from build123d import *

# Parameters (mm, degrees)
SKETCH2_W           = 12.139554842
SKETCH2_H           = 17.312906794
BOSS_EXTRUDE1_DEPTH = 15.24
SKETCH3_R           = 7.354852585
BOSS_EXTRUDE2_DEPTH = 1.27
SKETCH4_R           = 7.343962116
BOSS_EXTRUDE3_DEPTH = 19.05
FILLET1_R           = 5.08
FILLET2_R           = 2.54
SKETCH5_R           = 2.9177626
BOSS_EXTRUDE4_DEPTH = 13.97
BOSS_EXTRUDE5_DEPTH = 3.81
FILLET3_R           = 2.54
SKETCH8_R           = 1.866604038
CUT_EXTRUDE1_DEPTH  = 54.61
FILLET4_R           = 2.54


with BuildPart() as part:
    # Sketch1 → Revolve1 (revolve)
    with BuildSketch(Plane(origin=(0, 0, 0), x_dir=(1, 0, 0), z_dir=(0, 1, 0))):
        Polygon((0, 0), (-25.668765954, 0), (-37.871949768, 49.023134977), (-35.374465572, 49.023134977), (-23.974578156, 3.227035533), (0, 3.227035533), align=None)
    revolve(axis=Axis((0, 0, -3.227035533), (0, 0, 1)))

    # Sketch2 → Boss-Extrude1 (add)
    with BuildSketch(Plane.XY):
        Rectangle(SKETCH2_W, SKETCH2_H)
    extrude(amount=BOSS_EXTRUDE1_DEPTH)

    # Sketch3 → Boss-Extrude2 (add)
    with BuildSketch(Plane(origin=(0, 8.656453397, 0), x_dir=(1, 0, 0), z_dir=(0, 1, 0))):
        with Locations((0, -6.679713392)):
            Circle(SKETCH3_R)
    extrude(amount=BOSS_EXTRUDE2_DEPTH)

    # Sketch4 → Boss-Extrude3 (add)
    with BuildSketch(Plane.XZ.offset(-8.656453397)):
        with Locations((0.010679396, 6.67757966)):
            Circle(SKETCH4_R)
    extrude(amount=BOSS_EXTRUDE3_DEPTH)

    # Fillet1
    fillet1_edges = [part.edges().sort_by_distance(p)[0] for p in [
        (23.974578156, 0, -3.227035533),
    ]]
    fillet(fillet1_edges, radius=FILLET1_R)

    # Fillet2
    fillet2_edges = [part.edges().sort_by_distance(p)[0] for p in [
        (25.668765954, 0, 0),
    ]]
    fillet(fillet2_edges, radius=FILLET2_R)

    # Sketch5 → Boss-Extrude4 (add)
    with BuildSketch(Plane.XY.offset(15.24)):
        Circle(SKETCH5_R)
    extrude(amount=BOSS_EXTRUDE4_DEPTH)

    # Sketch6 → Boss-Extrude5 (add)
    with BuildSketch(Plane.XY.offset(15.24)):
        Polygon((1.022367717, -3.695378883), (3.711475848, -0.962293026), (2.689108131, 2.733085857), (-1.022367717, 3.695378883), (-3.711475848, 0.962293026), (-2.689108131, -2.733085857), align=None)
    extrude(amount=BOSS_EXTRUDE5_DEPTH)

    # Fillet3
    # the kernel refuses this fillet: 2.54 mm, written as the material it adds along each edge
    with BuildSketch(Plane(origin=(6.069777421, -8.656453397, 2.527747051), x_dir=(0, 0, -1), z_dir=(0, 1, 0))) as fillet3_piece_1:
        with BuildLine():
            CenterArc((0.723381963, -2.54), FILLET3_R, 90, 29.540761072)
            ThreePointArc((-0.52894629, -0.330186898), (-0.260967221, -0.170709801), (0, 0))
            Line((0, 0), (0.723381963, 0))
        make_face()
    extrude(amount=17.312906794)
    with BuildSketch(Plane(origin=(6.069777421, -8.656453397, 10.827412269), x_dir=(0.5295323324681384, 0, -0.8482897552551564), z_dir=(0, 1, 0))) as fillet3_piece_2:
        with BuildLine():
            CenterArc((0.731374616, -2.537710116), FILLET3_R, 92.433100789, 29.540761072)
            Line((-0.613637508, -0.383054138), (0, 0))
            ThreePointArc((0, 0), (0.311772179, -0.006620794), (0.623544358, 0))
        make_face()
    extrude(amount=17.312906794)
    with BuildSketch(Plane(origin=(-6.069777421, -8.656453397, 10.796053219), x_dir=(-0.5254687488151466, 0, -0.8508129018877444), z_dir=(0, 1, 0))) as fillet3_piece_3:
        with BuildLine():
            CenterArc((0.724778579, 2.537751252), FILLET3_R, 238.300195445, 29.288660156)
            Line((-0.609912043, 0.376686481), (0, 0))
            ThreePointArc((0, 0), (0.308960404, 0.006501859), (0.617920808, 0))
        make_face()
    extrude(amount=17.312906794)
    with BuildSketch(Plane(origin=(-6.069777421, -8.656453397, 2.559106101), x_dir=(-0.5254687488151472, 0, 0.8508129018877438), z_dir=(0, 1, 0))) as fillet3_piece_4:
        with BuildLine():
            CenterArc((0.724778579, -2.537751252), FILLET3_R, 92.411144399, 29.288660156)
            Line((-0.609912043, -0.376686481), (0, 0))
            ThreePointArc((0, 0), (0.308960404, -0.006501859), (0.617920808, 0))
        make_face()
    extrude(amount=17.312906794)

    # Sketch8 → Cut-Extrude1 (cut)
    with BuildSketch(Plane(origin=(0, 0, -3.227035533), x_dir=(-1, 0, 0), z_dir=(0, 0, -1))):
        Circle(SKETCH8_R)
    extrude(amount=-CUT_EXTRUDE1_DEPTH, mode=Mode.SUBTRACT)

    # Fillet4
    fillet4_edges = [part.edges().sort_by_distance(p)[0] for p in [
        (1.866604038, 0, -3.227035533),
    ]]
    fillet(fillet4_edges, radius=FILLET4_R)


solid = part.part
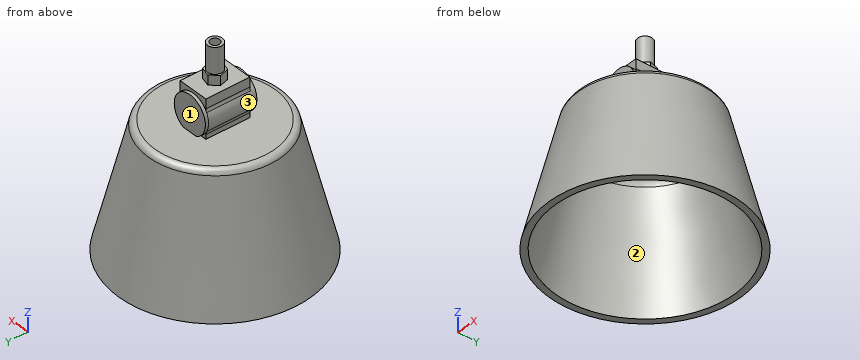
Could you check a few things on this model? Use its own coordinates, in mm. Face numbers are marked on the shaded views. Round coordinates to 2 decimals unless told otherwise and drop trailing zeros. Write each loop counter-clockwise with the first axis right and the second up, starting at its lowest first coordinate (ties: lowest second). Pieces come first, ordered by that corner, then holes. Notation, with made-up numbers: (0, -16.75) - (18, -16.75) arc R35 cw to (18, 17.25) - close; hole circle Ø11 at (89, -15.75). An arc over 180 degrees is marked (long way). Put each result on its own line as item: value. Start each with the question number.
(1) I need wall thicknesses on probe 1 along Y at (x, z) = (0, 7); probe 2 along Z at (x, y) = (-1, -11); probe 3 along Y at (x, z) = (-25, -23.5). Which ranges of each line are inside material? Lowest first, please.
(2) Thinking about a two-plate mould opening in Z: for the marked faces 1, 2 and 3, which applies, released by +Z, released by -Z, zero draft, split by the parting line, or undercut?
(3) Will these pins go through, and if not, where does the flat tip stop? pin 1 (1.5 mm diameter, centred on y = -5.5, z = 7.5, fed in from +X); pin 2 (4.5 mm diameter, centred on x = 0, y = 0, fed in from -Z); pin 3 (0.7 mm diameter, centred on x = 6.5, z = 4, fed in from -Y).
(4) I want a section at A-A, the plane z = -13.5. Please give me the cut outline in (x, y), plus the area to 3 significant figures.
Here are the results:
1. probe 1: y = -10.39 to -1.87, 1.87 to 9.93
1. probe 2: z = -3.23 to 0
1. probe 3: y = -19.19 to -14.74, 14.74 to 19.19
2. face 1: zero draft
2. face 2: released by -Z
2. face 3: undercut
3. pin 1: stops at x = 7.35
3. pin 2: stops at z = -2.03
3. pin 3: stops at y = -10.39
4. outline: circle Ø58.06 at (0, 0); hole circle Ø53.06 at (0, 0)
4. area: 436 mm^2
